Verification items for this drawing (mm, ordinates from the low corner). A direction names the side the tool comes from. Round coordinates to 2 decimals unless told otherwise and drop trailing zeros. Loops run counter-clockwise (first coordinate to the right, second up) from the corner with the lowest first, then second, coordinate; pieces in that order, holes last. Notation, with made-up numbers: (26.25, 55) -> (31.25, 55) arc R22 ccw to (31.25, 74) -> close; hole circle Ø7 at (19, 42.25). An arc over 180 degrees is marked (long way). Use a Markdown table: item, result. Add a question column.
Q1. Sectioned sample at B-B, the plane x = 9.5. Enter the section's corners in (y, z) (3 decimals), then the cut area to 3 significant figures.
Q2. Set-up check for the marked faces 1 and 2: record each of +Z, -Z, +X, -X, +Y, -Y from which the full face is reachable in a straight line by a thin tool's end or side.
Q3. Sectioned sample at C-C, the plane y = 23. Enter the section's corners in (x, z) (3 decimals), then the cut area to 3 significant figures.
Q4. Sectioned sample at D-D, the plane z = 28.5. Enter the section's corners in (x, y) (3 decimals).
Q5. Material ranges on L1, parallel to Y at x = 20, z = 47.5 (3 decimals), recorded low to high.
Q6. Gauge pin test, flat ends, axial feed: P1, Ø5, axis at x = 4.5, z = 34.5, coming from the +Y side; P2, Ø10, axis at x = 13.5, z = 10.5, coming from the +Y side (3 decimals); P3, Ø14.5, axis at y = 31.5, z = 23.5, coming from the +X side (3 decimals). Record the tip position at first contact, or that the pin passes through.
Q7. Sectioned sample at A-A, the plane z = 15. Enter the section's corners in (x, y) (3 decimals), then the cut area to 3 significant figures.
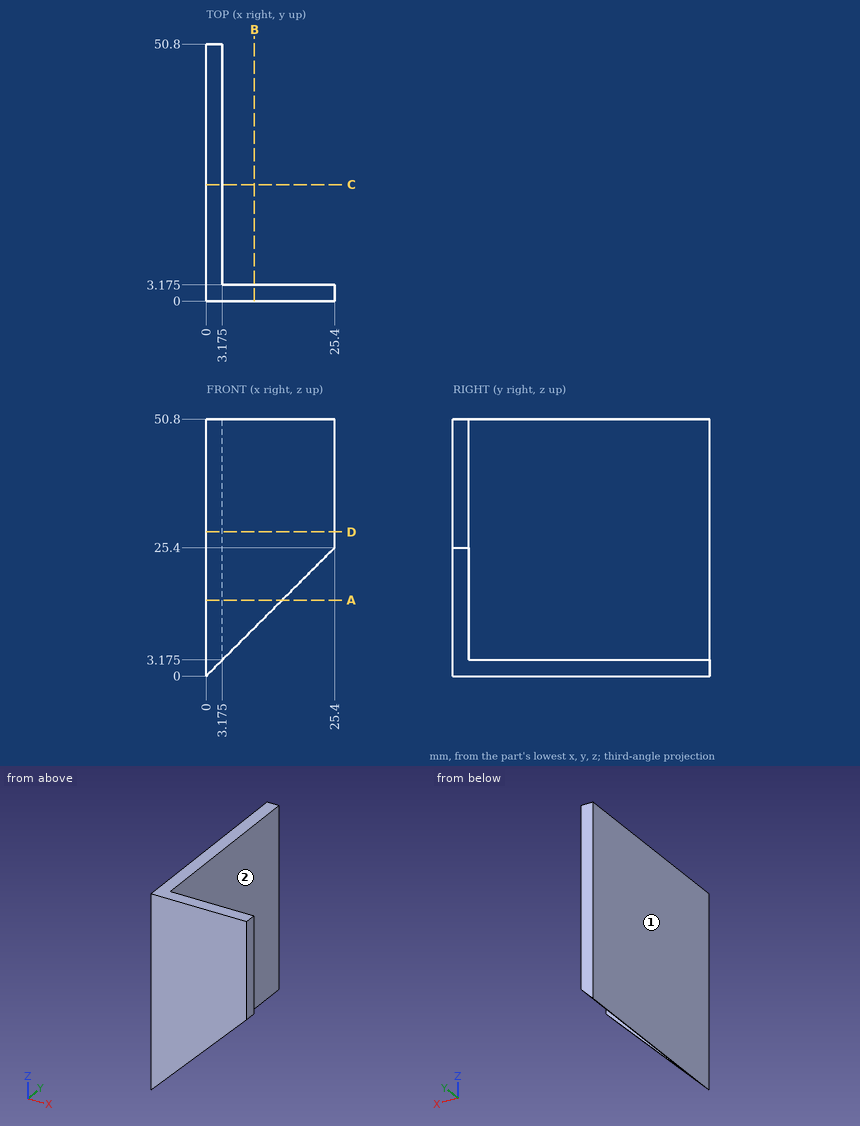
Values:
| question | item | result |
|---|---|---|
| 1 | outline | (0, 9.5) -> (3.175, 9.5) -> (3.175, 50.8) -> (0, 50.8) -> close |
| 1 | area | 131 mm^2 |
| 2 | face 1 | +Z, -Z, -X, +Y, -Y |
| 2 | face 2 | +Z, -Z, +X, +Y |
| 3 | outline | (0, 0) -> (3.175, 3.175) -> (3.175, 50.8) -> (0, 50.8) -> close |
| 3 | area | 156 mm^2 |
| 4 | outline | (0, 0) -> (25.4, 0) -> (25.4, 3.175) -> (3.175, 3.175) -> (3.175, 50.8) -> (0, 50.8) -> close |
| 5 | L1 | 0 to 3.175 |
| 6 | P1 | y = 50.8 |
| 6 | P2 | y = 3.175 |
| 6 | P3 | x = 3.175 |
| 7 | outline | (0, 0) -> (15, 0) -> (15, 3.175) -> (3.175, 3.175) -> (3.175, 50.8) -> (0, 50.8) -> close |
| 7 | area | 199 mm^2 |
